```python
from build123d import *

# Parameters (mm, degrees)
BOSS_EXTRUDE1_DEPTH = 2.54
BOSS_EXTRUDE2_START = -2.54
SKETCH1_3_R         = 1.5875
BOSS_EXTRUDE2_DEPTH = 2.54
CHAMFER1_SIZE       = 0.381
FILLET1_R           = 1.5875


with BuildPart() as part:
    # Sketch1 → Boss-Extrude1 (new body)
    with BuildSketch(Plane.XY):
        with BuildLine():
            Line((5.08, -28.575), (5.08, 0))
            ThreePointArc((5.08, 0), (0, 5.08), (-5.08, 0))
            Line((-5.08, 0), (-5.08, -28.575))
            ThreePointArc((-5.08, -28.575), (-4.15006403, -30.82006403), (-1.905, -31.75))
            Line((-1.905, -31.75), (1.905, -31.75))
            ThreePointArc((1.905, -31.75), (4.15006403, -30.82006403), (5.08, -28.575))
        make_face()
        with BuildLine():
            Line((-3.535704427, -0.30033797), (-2.190548714, -16.136074647))
            ThreePointArc((-2.190548714, -16.136074647), (-1.487288465, -17.568981304), (0, -18.1484375))
            ThreePointArc((0, -18.1484375), (1.487288465, -17.568981304), (2.190548714, -16.136074647))
            Line((2.190548714, -16.136074647), (3.535704427, -0.30033797))
            ThreePointArc((3.535704427, -0.30033797), (0, 3.5484375), (-3.535704427, -0.30033797))
        make_face(mode=Mode.SUBTRACT)
    extrude(amount=BOSS_EXTRUDE1_DEPTH)

    # Sketch1<3> → Boss-Extrude2 (add)
    with BuildSketch(Plane.XY.offset(BOSS_EXTRUDE2_START)):
        with BuildLine():
            ThreePointArc((1.905, -31.75), (4.15006403, -30.82006403), (5.08, -28.575))
            Line((5.08, -28.575), (5.08, 0))
            ThreePointArc((5.08, 0), (0, 5.08), (-5.08, 0))
            Line((-5.08, 0), (-5.08, -28.575))
            ThreePointArc((-5.08, -28.575), (-4.15006403, -30.82006403), (-1.905, -31.75))
            Line((-1.905, -31.75), (1.905, -31.75))
        make_face()
        Circle(SKETCH1_3_R, mode=Mode.SUBTRACT)
    extrude(amount=BOSS_EXTRUDE2_DEPTH)

    # Chamfer1
    chamfer1_edges = [part.edges().sort_by_distance(p)[0] for p in [
        (0, 3.5484375, 2.54),
        (2.86312657, -8.218206309, 2.54),
        (0, -18.1484375, 2.54),
        (-2.86312657, -8.218206309, 2.54),
    ]]
    chamfer(chamfer1_edges, length=CHAMFER1_SIZE)

    # Fillet1
    # the kernel refuses this fillet: 1.5875 mm, written as the material it takes off along each edge
    with BuildSketch(Plane(origin=(1.905, -28.575, 2.54), x_dir=(0, -1, 0), z_dir=(-1, 0, 0))) as fillet1_piece_1:
        with BuildLine():
            CenterArc((3.175 - FILLET1_R, -FILLET1_R), FILLET1_R, 0, 90)
            Line((3.175, -FILLET1_R), (3.175, 0))
            Line((3.175, 0), (3.175 - FILLET1_R, 0))
        make_face()
    revolve(axis=Axis((1.905, -28.575, 2.54), (0, 0, 1)), revolution_arc=90, mode=Mode.SUBTRACT)
    with BuildSketch(Plane(origin=(-1.905, -28.575, 2.54), x_dir=(-1, 0, 0), z_dir=(0, 1, 0))) as fillet1_piece_2:
        with BuildLine():
            CenterArc((3.175 - FILLET1_R, -FILLET1_R), FILLET1_R, 0, 90)
            Line((3.175, -FILLET1_R), (3.175, 0))
            Line((3.175, 0), (3.175 - FILLET1_R, 0))
        make_face()
    revolve(axis=Axis((-1.905, -28.575, 2.54), (0, 0, 1)), revolution_arc=90, mode=Mode.SUBTRACT)
    with BuildSketch(Plane(origin=(-5.08, 0, 2.54), x_dir=(1, 0, 0), z_dir=(0, -1, 0)), Plane(origin=(-5.08, 0, -2.54), x_dir=(0, 0, 1), z_dir=(0, -1, 0)), Plane(origin=(5.08, -28.575, 2.54), x_dir=(-1, 0, 0), z_dir=(0, 1, 0)), Plane(origin=(5.08, -28.575, -2.54), x_dir=(0, 0, 1), z_dir=(0, 1, 0))) as fillet1_piece_3:
        with BuildLine():
            CenterArc((FILLET1_R, -FILLET1_R), FILLET1_R, 90, 90)
            Line((0, -FILLET1_R), (0, 0))
            Line((0, 0), (FILLET1_R, 0))
        make_face()
    extrude(amount=28.575, mode=Mode.SUBTRACT)
    with BuildSketch(Plane(origin=(1.905, -28.575, -2.54), x_dir=(0, -1, 0), z_dir=(-1, 0, 0))) as fillet1_piece_4:
        with BuildLine():
            CenterArc((3.175 - FILLET1_R, FILLET1_R), FILLET1_R, 270, 90)
            Line((3.175 - FILLET1_R, 0), (3.175, 0))
            Line((3.175, 0), (3.175, FILLET1_R))
        make_face()
    revolve(axis=Axis((1.905, -28.575, -2.54), (0, 0, 1)), revolution_arc=90, mode=Mode.SUBTRACT)
    with BuildSketch(Plane(origin=(-1.905, -28.575, -2.54), x_dir=(-1, 0, 0), z_dir=(0, 1, 0))) as fillet1_piece_5:
        with BuildLine():
            CenterArc((3.175 - FILLET1_R, FILLET1_R), FILLET1_R, 270, 90)
            Line((3.175 - FILLET1_R, 0), (3.175, 0))
            Line((3.175, 0), (3.175, FILLET1_R))
        make_face()
    revolve(axis=Axis((-1.905, -28.575, -2.54), (0, 0, 1)), revolution_arc=90, mode=Mode.SUBTRACT)
    with BuildSketch(Plane(origin=(0, 0, -2.54), x_dir=(1, 0, 0), z_dir=(0, -1, 0))) as fillet1_piece_6:
        with BuildLine():
            CenterArc((5.08 - FILLET1_R, FILLET1_R), FILLET1_R, 270, 90)
            Line((5.08 - FILLET1_R, 0), (5.08, 0))
            Line((5.08, 0), (5.08, FILLET1_R))
        make_face()
    revolve(axis=Axis((0, 0, -2.54), (0, 0, 1)), revolution_arc=180, mode=Mode.SUBTRACT)
    with BuildSketch(Plane(origin=(0, 0, 2.54), x_dir=(1, 0, 0), z_dir=(0, -1, 0))) as fillet1_piece_7:
        with BuildLine():
            CenterArc((5.08 - FILLET1_R, -FILLET1_R), FILLET1_R, 0, 90)
            Line((5.08, -FILLET1_R), (5.08, 0))
            Line((5.08, 0), (5.08 - FILLET1_R, 0))
        make_face()
    revolve(axis=Axis((0, 0, 2.54), (0, 0, 1)), revolution_arc=180, mode=Mode.SUBTRACT)
    with BuildSketch(Plane(origin=(-1.905, -31.75, 2.54), x_dir=(0, 1, 0), z_dir=(1, 0, 0)), Plane(origin=(-1.905, -31.75, -2.54), x_dir=(0, 0, 1), z_dir=(1, 0, 0))) as fillet1_piece_8:
        with BuildLine():
            CenterArc((FILLET1_R, -FILLET1_R), FILLET1_R, 90, 90)
            Line((0, -FILLET1_R), (0, 0))
            Line((0, 0), (FILLET1_R, 0))
        make_face()
    extrude(amount=3.81, mode=Mode.SUBTRACT)


solid = part.part
```
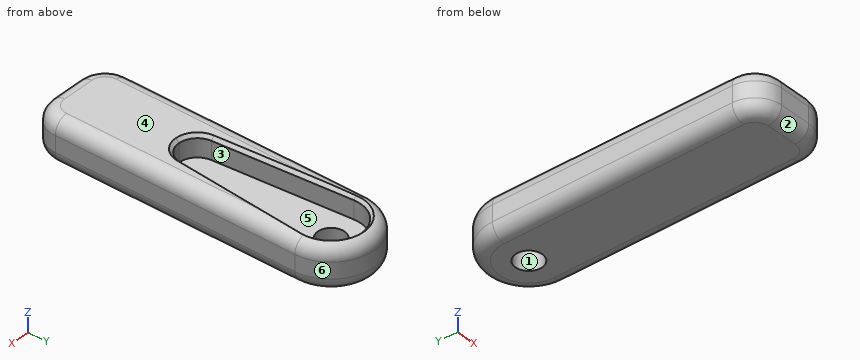
The listing builds one solid part. Answer for the finished solid, in the listing's coordinates (mm). Face numbers are marked on the shaded views. A direction names the side the tool comes from. Give positions to 0.01 mm unless a question says otherwise; leave off trailing zeros. Loops run counter-clockwise (first coordinate to the right, second up) from the corner with the lowest first, then second, coordinate; pieces in that order, holes last. Notation, with made-up numbers: M 21.5,55.25 L 43.5,55.25 A25 cw 43.5,87.25 Z; hole C 79,12.25 d4. An arc over 180 degrees is marked long. One line per item, written item: value.
Q1. Find the intervals of material crossed by line 1 (Y direction, x = 0, z = 0.6); line 2 (Y direction, x = 0, z = -0.35); line 3 (Z direction, x = -1.75, y = -9), in increasing order. Write a range as from..to.
Working result:
line 1: y = -31.75..-18.15, 3.55..5.08
line 2: y = -31.75..-1.59, 1.59..5.08
line 3: z = -2.54..0
Q2. A flat-ended cylindrical pin translates along its axis: P1, Ø1, axis at x = -0.5, y = -17, coming from the +Z side. Find the tip coordinate at first contact, or state that the pin passes through.
Working result:
P1: stops at z = 0
Q3. Determine the mould class of the marked faces 1, 2, 3 and 4 for opening direction Y: +Y half, -Y half, draft (parallel to the pull), parting line (faces both ways), or undercut.
Working result:
face 1: undercut
face 2: -Y half
face 3: undercut
face 4: draft
Q4. A cutting plane is placed at C-C on y = -12. Determine the outline of the cut face in (x, z) (1 decimal), then the cut area to 3 significant figures.
Working result:
outline: M -5.1,-1 A1.6 ccw -3.5,-2.5 L 3.5,-2.5 A1.6 ccw 5.1,-1 L 5.1,1 A1.6 ccw 3.5,2.5 L 2.9,2.5 L 2.5,2.2 L 2.5,0 L -2.5,0 L -2.5,2.2 L -2.9,2.5 L -3.5,2.5 A1.6 ccw -5.1,1 Z
area: 36.4 mm^2
Q5. A cutting plane is placed at A-A on y = -1. Determine the outline of the cut face in (x, z) (1 decimal).
Working result:
outline: M -5.1,-1 A1.6 ccw -3.5,-2.5 L -1.2,-2.5 L -1.2,0 L -3.5,0 L -3.5,2.2 L -3.8,2.5 A1.6 ccw -5.1,1 Z; M 1.2,-2.5 L 3.5,-2.5 A1.6 ccw 5.1,-1 L 5.1,1 A1.6 ccw 3.8,2.5 L 3.5,2.2 L 3.5,0 L 1.2,0 Z
Q6. For the marked faces 5 and 6, determine the directions among +Z, -Z, +X, -X, +Y, -Y from which every point of the face is accessible in a straight line to the end or side of a thin tool.
Working result:
face 5: +Z
face 6: +Z, -Z, +Y
